```python
from build123d import *

# Parameters (mm, degrees)
BOSS_EXTRUDE1_DEPTH = 6.35
SKETCH2_R           = 0.62000003
CUT_EXTRUDE1_DEPTH  = 6.35
SKETCH3_R           = 2.480100005
CUT_EXTRUDE2_DEPTH  = 6.35


with BuildPart() as part:
    # Sketch1 → Boss-Extrude1 (new body)
    with BuildSketch(Plane(origin=(0, 0, 0), x_dir=(1, 0, 0), z_dir=(0, 1, 0))):
        with BuildLine():
            Line((-25.4, 0), (-25.4, -88.9))
            Line((-25.4, -88.9), (25.4, -88.9))
            Line((25.4, -88.9), (25.4, 0))
            ThreePointArc((25.4, 0), (0, 25.4), (-25.4, 0))
        make_face()
    extrude(amount=BOSS_EXTRUDE1_DEPTH)

    # Sketch2 → Cut-Extrude1 (cut)
    with BuildSketch(Plane(origin=(0, 6.35, 0), x_dir=(1, 0, 0), z_dir=(0, 1, 0))):
        with Locations(Location((0, 13.271000001, 0), (0, 0, 270))):
            Circle(SKETCH2_R)
        with Locations(Location((0, -13.271000001, 0), (0, 0, 270))):
            Circle(SKETCH2_R)
        with Locations(Location((-11.493023134, 6.635500001, 0), (0, 0, 270))):
            Circle(SKETCH2_R)
        with Locations(Location((-11.493023134, -6.635500001, 0), (0, 0, 270))):
            Circle(SKETCH2_R)
        with Locations(Location((11.493023134, 6.635500001, 0), (0, 0, 270))):
            Circle(SKETCH2_R)
        with Locations(Location((11.493023134, -6.635500001, 0), (0, 0, 270))):
            Circle(SKETCH2_R)
    extrude(amount=-CUT_EXTRUDE1_DEPTH, mode=Mode.SUBTRACT)

    # Sketch3 → Cut-Extrude2 (cut)
    with BuildSketch(Plane(origin=(0, 6.35, 0), x_dir=(1, 0, 0), z_dir=(0, 1, 0))):
        with Locations(Location((0, 0, 0), (0, 0, 270))):
            Circle(SKETCH3_R)
    extrude(amount=-CUT_EXTRUDE2_DEPTH, mode=Mode.SUBTRACT)


solid = part.part
```
The model under review builds one solid part; all positions refer to its coordinate system, in mm. Round coordinates to 2 decimals unless told otherwise and drop trailing zeros. Order: outer loops, then holes, each group sorted by start corner. A loop starts at its lowest first (then second) coordinate and runs counter-clockwise, first axis right, second up. Notation, with made-up numbers: (87, 56) - (126, 56) arc R27 cw to (126, 95) - close; hole circle Ø2 at (82, -36.75). An arc over 180 degrees is marked (long way). Answer in a Markdown table with one row per item.
(1) Take a section at C-C on z = -10.5. Write out the cut boundary in (x, y).
Result set:
| item | result |
|---|---|
| outline | (-23.13, 0) - (23.13, 0) - (23.13, 6.35) - (-23.13, 6.35) - close |
(2) Clearance check with flat-ended pins moving along their axes: P1, Ø2, axis at x = -4, y = 1, coming from the -Z side; P2, Ø2, axis at x = 19.5, y = 1, coming from the -Z side. State where each tip first meets the part, or that it passes through.
Result set:
| item | result |
|---|---|
| P1 | stops at z = -25.22 |
| P2 | stops at z = -17.4 |
(3) Take a section at A-A on y = 2.5. Write out the cut boundary in (x, z).
Result set:
| item | result |
|---|---|
| outline | (-25.4, 0) arc R25.4 ccw to (25.4, 0) - (25.4, 88.9) - (-25.4, 88.9) - close; hole circle Ø1.24 at (-11.49, -6.64); hole circle Ø1.24 at (-11.49, 6.64); hole circle Ø4.96 at (0, 0); hole circle Ø1.24 at (0, -13.27); hole circle Ø1.24 at (0, 13.27); hole circle Ø1.24 at (11.49, -6.64); hole circle Ø1.24 at (11.49, 6.64) |
(4) Take a section at B-B on x = 16.5. Write out the cut boundary in (y, z).
Result set:
| item | result |
|---|---|
| outline | (0, -19.31) - (6.35, -19.31) - (6.35, 88.9) - (0, 88.9) - close |
(5) Mouldability with a two-part tool opening along Z and no side actions: class faces 1 (the face through (0.559, 3.131, -25.394)), 2 (the face through (0.745, 3.219, 2.366)), 3 (the face through (0, 3, 88.9)), 4 (the face through (0, 6.35, 31)) as released by +Z, released by -Z, zero draft, split by the parting line, or undercut.
Result set:
| item | result |
|---|---|
| face 1 | released by -Z |
| face 2 | undercut |
| face 3 | released by +Z |
| face 4 | zero draft |
(6) For line 1 (X direction, y = 0.75, z = 13); line 2 (Z direction, x = 20, y = 3.5); line 3 (Z direction, x = -6, y = 1.25), list the stretches that pass through material, from the lowest coordinate up. Write a range as from..to.
Result set:
| item | result |
|---|---|
| line 1 | x = -25.4..-0.56, 0.56..25.4 |
| line 2 | z = -15.66..88.9 |
| line 3 | z = -24.68..88.9 |
